Geometry check sheet. Reference: drawing and pictorial views, mm from the part's lowest x, y, z. Give positions to 0.01 mm unless a question says otherwise; leave off trailing zeros. Write each loop counter-clockwise with the first axis right and the second up, starting at its lowest first coordinate (ties: lowest second). Pieces come first, ordered by that corner, then holes. Notation, with made-up numbers: (48.25, 22.25) -> (72.25, 22.25) arc R21 ccw to (72.25, 51.25) -> close; hole circle Ø5 at (20.5, 13.25). An arc over 180 degrees is marked (long way). Answer as CSV lines item,"result".
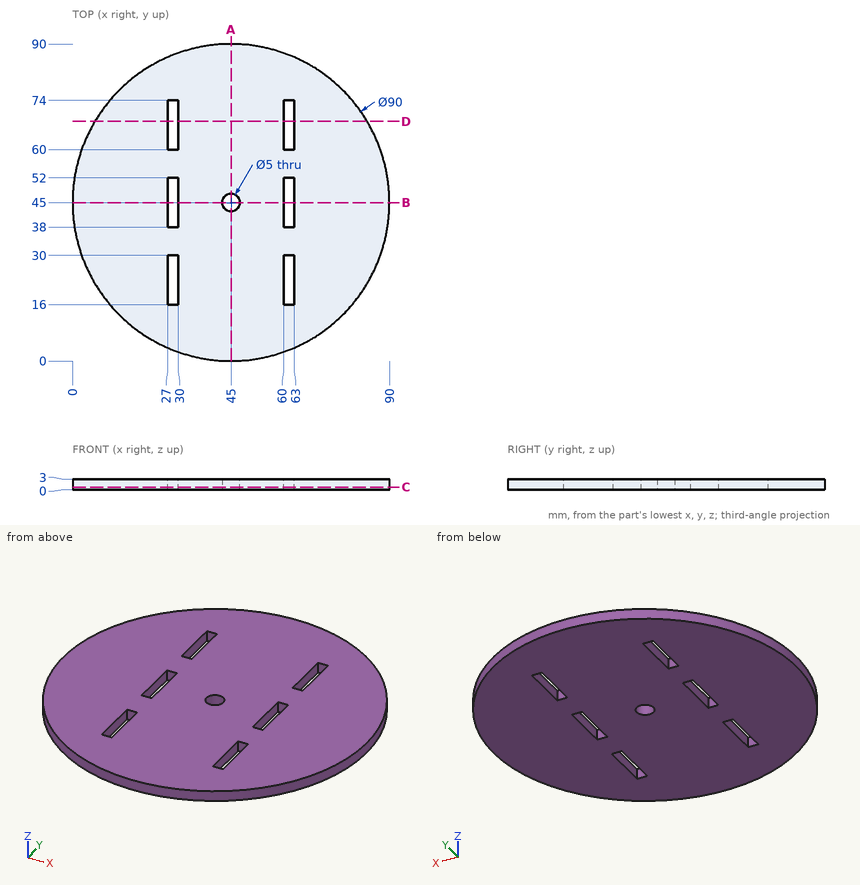
1) Section check D-D (y = 68). Record the boundary of the cut face in (x, z).
Reported:
outline,"(6.32, 0) -> (27, 0) -> (27, 3) -> (6.32, 3) -> close; (30, 0) -> (60, 0) -> (60, 3) -> (30, 3) -> close; (63, 0) -> (83.68, 0) -> (83.68, 3) -> (63, 3) -> close"
2) Section check C-C (z = 0.7). Record the boundary of the cut face in (x, y), and give its area (3 significant figures).
Reported:
outline,"circle Ø90 at (45, 45); hole (27, 16) -> (30, 16) -> (30, 30) -> (27, 30) -> close; hole (27, 38) -> (30, 38) -> (30, 52) -> (27, 52) -> close; hole (27, 60) -> (30, 60) -> (30, 74) -> (27, 74) -> close; hole circle Ø5 at (45, 45); hole (60, 16) -> (63, 16) -> (63, 30) -> (60, 30) -> close; hole (60, 38) -> (63, 38) -> (63, 52) -> (60, 52) -> close; hole (60, 60) -> (63, 60) -> (63, 74) -> (60, 74) -> close"
area,"6,090 mm²"
3) Scan lines: line 1 along Y through (x, z) = (45, 1.5); line 2 along X through (y, z) = (19, 2.15); line 3 along X through (y, z) = (64.5, 2.2). Record each from-to range of solid material in increasing order.
Reported:
line 1,"0 to 42.5, 47.5 to 90"
line 2,"8.27 to 27, 30 to 60, 63 to 81.73"
line 3,"4.44 to 27, 30 to 60, 63 to 85.56"
4) Depth check by flat-ended pin: pin 1 (1.5 mm diameter, centred on x = 28.5, z = 2, fed in from -Y); pin 2 (5 mm diameter, centred on x = 13, y = 73, fed in from -Z); pin 3 (1.5 mm diameter, centred on y = 44, z = 1.5, fed in from +X); pin 4 (1.5 mm diameter, centred on y = 23.5, z = 1.5, fed in from -X). Enter the tip coordinate at first touch or a pass-through.
Reported:
pin 1,"y = 2.85"
pin 2,"z = 0"
pin 3,"x = 90"
pin 4,"x = 5.07"
5) Section check A-A (x = 45). Record the boundary of the cut face in (y, z), and give its area (3 significant figures).
Reported:
outline,"(0, 0) -> (42.5, 0) -> (42.5, 3) -> (0, 3) -> close; (47.5, 0) -> (90, 0) -> (90, 3) -> (47.5, 3) -> close"
area,"255 mm²"
6) Section check B-B (y = 45). Record the boundary of the cut face in (x, z), and give its area (3 significant figures).
Reported:
outline,"(0, 0) -> (27, 0) -> (27, 3) -> (0, 3) -> close; (30, 0) -> (42.5, 0) -> (42.5, 3) -> (30, 3) -> close; (47.5, 0) -> (60, 0) -> (60, 3) -> (47.5, 3) -> close; (63, 0) -> (90, 0) -> (90, 3) -> (63, 3) -> close"
area,"237 mm²"
